```python
from build123d import *

# Parameters (mm, degrees)
S01_TURNED_STEEL_BODY_R               = 8
F_01_TURNED_STEEL_BODY_DEPTH          = 52
F_02_START                            = -2.5
S02_BACKPLATE_LOCATING_SPIGOT_R       = 5
F_02_BACKPLATE_LOCATING_SPIGOT_DEPTH  = 2.5
F_03_START                            = 52
S03_TRACK_LOCATING_SPIGOT_R           = 5
F_03_TRACK_LOCATING_SPIGOT_DEPTH      = 1.25
F_04_START                            = -2.6
S04_REAR_M6_THREADED_ENVELOPE_R       = 3.03
F_04_REAR_M6_THREADED_ENVELOPE_DEPTH  = 14.1
F_05_START                            = 38.5
S05_FRONT_M6_THREADED_ENVELOPE_R      = 3.03
F_05_FRONT_M6_THREADED_ENVELOPE_DEPTH = 15


with BuildPart() as part:
    # S01 - Turned steel body → 01 - Turned steel body (new body)
    with BuildSketch(Plane.XY):
        Circle(S01_TURNED_STEEL_BODY_R)
    extrude(amount=F_01_TURNED_STEEL_BODY_DEPTH)

    # S02 - Backplate locating spigot → 02 - Backplate locating spigot (add)
    with BuildSketch(Plane.XY.offset(F_02_START)):
        Circle(S02_BACKPLATE_LOCATING_SPIGOT_R)
    extrude(amount=F_02_BACKPLATE_LOCATING_SPIGOT_DEPTH)

    # S03 - Track locating spigot → 03 - Track locating spigot (add)
    with BuildSketch(Plane.XY.offset(F_03_START)):
        Circle(S03_TRACK_LOCATING_SPIGOT_R)
    extrude(amount=F_03_TRACK_LOCATING_SPIGOT_DEPTH)

    # S04 - Rear M6 threaded envelope → 04 - Rear M6 threaded envelope (cut)
    with BuildSketch(Plane.XY.offset(F_04_START)):
        Circle(S04_REAR_M6_THREADED_ENVELOPE_R)
    extrude(amount=F_04_REAR_M6_THREADED_ENVELOPE_DEPTH, mode=Mode.SUBTRACT)

    # S05 - Front M6 threaded envelope → 05 - Front M6 threaded envelope (cut)
    with BuildSketch(Plane.XY.offset(F_05_START)):
        Circle(S05_FRONT_M6_THREADED_ENVELOPE_R)
    extrude(amount=F_05_FRONT_M6_THREADED_ENVELOPE_DEPTH, mode=Mode.SUBTRACT)


solid = part.part
```
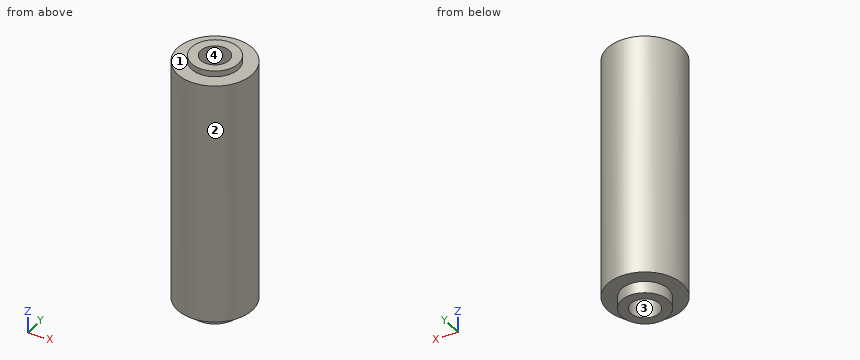
Design review of the part built by this model. Coordinates are the model's own, in mm. Face numbers are marked on the shaded views. Coordinates: 2 decimals unless noted, no trailing zeros. Order: outer loops, then holes, each group sorted by start corner. A loop starts at its lowest first (then second) coordinate and runs counter-clockwise, first axis right, second up. Notation, with made-up numbers: (46, 44) - (53, 44) arc R17 ccw to (53, 65) - close; hole circle Ø8 at (16, 84.5). An arc over 180 degrees is marked (long way). Answer in a Markdown table with one row per item.
(1) Wall thickness on line 1 along Y through (x, z) = (0, 43); line 2 along Z through (x, y) = (0, -1.5); line 3 along Z through (x, y) = (-3.5, 5): over which ranges is each line inside the solid? List them lowest first. Write a range as from..to.
Checked values:
| item | result |
|---|---|
| line 1 | -8..-3.03, 3.03..8 |
| line 2 | 11.5..38.5 |
| line 3 | 0..52 |
(2) Consider section D-D on z = 23.5. State the section outline as (x, y) points, plus the area to 3 significant figures.
Checked values:
| item | result |
|---|---|
| outline | circle Ø16 at (0, 0) |
| area | 201 mm^2 |
(3) Consider section B-B on x = 0. State the section outline as (y, z) points.
Checked values:
| item | result |
|---|---|
| outline | (-8, 0) - (-5, 0) - (-5, -2.5) - (-3.03, -2.5) - (-3.03, 11.5) - (3.03, 11.5) - (3.03, -2.5) - (5, -2.5) - (5, 0) - (8, 0) - (8, 52) - (5, 52) - (5, 53.25) - (3.03, 53.25) - (3.03, 38.5) - (-3.03, 38.5) - (-3.03, 53.25) - (-5, 53.25) - (-5, 52) - (-8, 52) - close |
(4) The part is to be moulded in two halves that separate along Y. For the marked faces 1, 2, 3 and 4, say which applies: released by +Y, released by -Y, zero draft, split by the parting line, or undercut.
Checked values:
| item | result |
|---|---|
| face 1 | zero draft |
| face 2 | split by the parting line |
| face 3 | undercut |
| face 4 | undercut |
(5) Clearance check with flat-ended pins moving along their axes: pin 1 (5 mm diameter, centred on x = 0, y = 0, fed in from +Z); pin 2 (1.5 mm diameter, centred on x = -4.5, z = 11, fed in from -Y); pin 3 (2 mm diameter, centred on y = -3, z = 22, fed in from -X). State where each tip first meets the part, or that it passes through.
Checked values:
| item | result |
|---|---|
| pin 1 | z = 38.5 |
| pin 2 | y = -7.07 |
| pin 3 | x = -7.75 |
(6) Consider section A-A on z = 7.5. State the section outline as (x, y) points, plus the area to 3 significant figures.
Checked values:
| item | result |
|---|---|
| outline | circle Ø16 at (0, 0); hole circle Ø6.06 at (0, 0) |
| area | 172 mm^2 |
